Work out the finished part from the listing and answer in its coordinate system (mm). A direction names the side the tool comes from. Give positions to 0.01 mm unless a question says otherwise; leave off trailing zeros. Write each loop counter-clockwise with the first axis right and the second up, starting at its lowest first coordinate (ties: lowest second). Pieces come first, ordered by that corner, then holes. Notation, with made-up numbers: (-9, -31.75) - (1, -31.75) arc R18 ccw to (1, -18.75) - close; hole circle Ø9 at (-25, 37.5). An arc over 180 degrees is marked (long way). Write item = value, one per line.
from build123d import *

# Parameters (mm, degrees)
SKETCH1_R            = 11.55
SKETCH1_R_2          = 8.55
BOSS_EXTRUDE1_DEPTH  = 5
SKETCH2_W            = 5
SKETCH2_H            = 23.723808267
BOSS_EXTRUDE2_DEPTH  = 5
BOSS_EXTRUDE3_DEPTH  = 5
FILLET1_R            = 1
SKETCH38_W           = 12
SKETCH38_H           = 3.5
BOSS_EXTRUDE28_DEPTH = 12
CUT_EXTRUDE3_REACH   = 49.704
SKETCH39_R           = 2.75
CHAMFER1_SIZE        = 2.5
FILLET3_R            = 1
SKETCH1_3_R          = 8.55
SKETCH1_3_R_2        = 7.25
BOSS_EXTRUDE29_DEPTH = 1


with BuildPart() as part:
    # Sketch1 → Boss-Extrude1 (new body)
    with BuildSketch(Plane(origin=(0, 0, 0), x_dir=(0, 0, -1), z_dir=(1, 0, 0))):
        Circle(SKETCH1_R)
        Circle(SKETCH1_R_2, mode=Mode.SUBTRACT)
    extrude(amount=-BOSS_EXTRUDE1_DEPTH)

    # Sketch2 → Boss-Extrude2 (add)
    with BuildSketch(Plane(origin=(0, 0, 0), x_dir=(0, 0, -1), z_dir=(1, 0, 0))):
        with Locations((0, -23.138095867)):
            Rectangle(SKETCH2_W, SKETCH2_H)
    extrude(amount=-BOSS_EXTRUDE2_DEPTH)

    # Sketch3 → Boss-Extrude3 (add)
    with BuildSketch(Plane(origin=(0, 0, 0), x_dir=(0, 0, -1), z_dir=(1, 0, 0))):
        Polygon((-9.5, -35), (-9.5, -34), (9.5, -34), (9.5, -35), (3.05, -35), (3.05, -37.4), (5.45, -37.4), (5.45, -38.4), (3.05, -40), (-3.05, -40), (-5.45, -38.4), (-5.45, -37.4), (-3.05, -37.4), (-3.05, -35), align=None)
    extrude(amount=-BOSS_EXTRUDE3_DEPTH)

    # Fillet1
    fillet1_edges = [part.edges().sort_by_distance(p)[0] for p in [
        (0, -37.9, 5.45),
        (0, -37.9, -5.45),
    ]]
    fillet(fillet1_edges, radius=FILLET1_R)

    # Sketch38 → Boss-Extrude28 (add)
    with BuildSketch(Plane.ZY.offset(5)):
        with Locations((0, -33.25)):
            Rectangle(SKETCH38_W, SKETCH38_H)
    extrude(amount=BOSS_EXTRUDE28_DEPTH)

    # Sketch39 → Cut-Extrude3 (cut, up to next)
    with BuildSketch(Plane(origin=(0, -31.5, 0), x_dir=(1, 0, 0), z_dir=(0, 1, 0)), mode=Mode.PRIVATE) as cut_extrude3_sk1:
        with Locations(Location((-11, 0, 0), (0, 0, 270))):
            Circle(SKETCH39_R)
    cut_extrude3_tool1 = extrude(cut_extrude3_sk1.sketch, amount=-CUT_EXTRUDE3_REACH, mode=Mode.PRIVATE) & part.part
    add(cut_extrude3_tool1.solids().sort_by_distance((-11, -31.5, 0))[0], mode=Mode.SUBTRACT)

    # Chamfer1
    chamfer1_edges = [part.edges().sort_by_distance(p)[0] for p in [
        (-5, -31.5, 4.25),
        (-5, -31.5, -4.25),
    ]]
    chamfer(chamfer1_edges, length=CHAMFER1_SIZE - 0.0001)  # a hair under: the kernel refuses the full size

    # Fillet3
    fillet3_edges = [part.edges().sort_by_distance(p)[0] for p in [
        (-5, 0, 8.55),
    ]]
    fillet(fillet3_edges, radius=FILLET3_R)

    # Sketch1<3> → Boss-Extrude29 (add)
    with BuildSketch(Plane(origin=(0, 0, 0), x_dir=(0, 0, -1), z_dir=(1, 0, 0))):
        Circle(SKETCH1_3_R)
        Circle(SKETCH1_3_R_2, mode=Mode.SUBTRACT)
    extrude(amount=-BOSS_EXTRUDE29_DEPTH)


solid = part.part
1. Straight lines are drawn through the part: line 1 (Y direction, x = -4.5, z = 7.25); line 2 (Y direction, x = -3.5, z = -6); line 3 (Y direction, x = -5.5, z = -0.75). For each, find the intervals that lie inside material, in ascending order.
Solution:
line_1 = -35 to -34, -8.99 to -4.78, 4.78 to 8.99
line_2 = -35 to -34, -9.87 to -6.09, 6.09 to 9.87
line_3 = -35 to -31.5
2. Find section C-C, the plane x = -11. Give the vertices of the cut face in (y, z), then the cut area to 4 significant figures.
Solution:
outline = (-35, -6) - (-31.5, -6) - (-31.5, -2.75) - (-35, -2.75) - close; (-35, 2.75) - (-31.5, 2.75) - (-31.5, 6) - (-35, 6) - close
area = 22.75 mm^2
3. For a pull along X with two mould halves and no side action, classify faces 1 (the flat face through (-6, -33, 4)), 2 (the cylindrical face through (-8.273, -33.226, -0.358)), 3 (the flat face through (-2, -34, -6)), 4 (the flat face through (-5, -37, 0)) as pulls with the +X half, pulls with the -X half, needs draft (parallel to the pull), parting line crosses it, or undercut.
Solution:
face_1 = pulls with the +X half
face_2 = undercut
face_3 = needs draft
face_4 = pulls with the -X half
4. Find section A-A, the plane z = 0. Give the vertices of the cut face in (x, y), then the cut area to 3 significant figures.
Solution:
outline = (-17, -35) - (-13.75, -35) - (-13.75, -31.5) - (-17, -31.5) - close; (-8.25, -35) - (-5, -35) - (-5, -40) - (0, -40) - (0, -7.25) - (-1, -7.25) - (-1, -8.55) - (-4, -8.55) arc R1 ccw to (-5, -9.55) - (-5, -31.5) - (-8.25, -31.5) - close; (-5, 9.55) arc R1 ccw to (-4, 8.55) - (-1, 8.55) - (-1, 7.25) - (0, 7.25) - (0, 11.55) - (-5, 11.55) - close
area = 197 mm^2
5. Find section B-B, the plane y = 0. Give the vertices of the cut face in (x, z).
Solution:
outline = (-5, -11.55) - (0, -11.55) - (0, -7.25) - (-1, -7.25) - (-1, -8.55) - (-4, -8.55) arc R1 ccw to (-5, -9.55) - close; (-5, 9.55) arc R1 ccw to (-4, 8.55) - (-1, 8.55) - (-1, 7.25) - (0, 7.25) - (0, 11.55) - (-5, 11.55) - close
6. A tool of negligible diameter and unlimited length cuts with its end or side. For faces 5 (the flat face through (-2.5, -34.5, -9.5)), 6 (the flat face through (-2, -34, 6)), 7 (the flat face through (-11, -33, 6)), from which of +Z, -Z, +X, -X, +Y, -Y can it reach the whole face along a straight path? Write none if from no direction.
Solution:
face_5 = -Z, +X, -X, -Y
face_6 = +Z, +X
face_7 = +Z, -X, +Y, -Y
7. Given pin 1 (4 mm diameter, centred on x = -7.5, y = -14.5, fed in from -Z); pin 2 (1.1 mm diameter, centred on x = -3, y = -34.5, fed in from +Z); pin 3 (3 mm diameter, centred on x = -3.5, z = 9, fed in from -Y); pin 4 (5.5 mm diameter, centred on y = -38, z = 2.5, fed in from -X), each flat-ended and moving along its own axis, determine where each tip first touches the part or whether it passes through.
Solution:
pin_1 = through
pin_2 = 9.5
pin_3 = -35
pin_4 = -5
8. Find section D-D, the plane y = -18. Give the vertices of the cut face in (x, z), then the cut area to 3 significant figures.
Solution:
outline = (-5, -2.5) - (0, -2.5) - (0, 2.5) - (-5, 2.5) - close
area = 25.0 mm^2
